from build123d import *

# Parameters (mm, degrees)
CUT_EXTRUDE_1_REACH = 10.022


with BuildPart() as part:
    # 草图1 → 旋转1 (revolve)
    with BuildSketch(Plane.XY, mode=Mode.PRIVATE) as revolve_1_sk:
        Polygon((1.5, -1.8), (1.5, -6.75), (1.25, -7), (0, -7), (0, -1.877350269), (1, -1.3), (1, 0), (2.77, 0), (2.77, -0.53), align=None)
    revolve(revolve_1_sk.sketch.rotate(Axis((0, 0, 0), (0, 1, 0)), 90), axis=Axis((0, 0, 0), (0, 1, 0)))

    # 切除-拉伸1: up to this cone (the profile starts inside it)
    cut_extrude_1_end = Plane(origin=(0, 0, 0), z_dir=(0, 1, 0)).offset(-1.877349269) * Cone(1.732e-06, 27.108355455, 15.651015319, align=(Align.CENTER, Align.CENTER, Align.MIN), mode=Mode.PRIVATE)
    # 草图2 → 切除-拉伸1 (cut, up to the surface)
    with BuildSketch(Plane(origin=(0, 0, 0), x_dir=(1, 0, 0), z_dir=(0, 1, 0)), mode=Mode.PRIVATE) as cut_extrude_1_sk1:
        Polygon((1.154700538, 0), (0.577350269, 1), (-0.577350269, 1), (-1.154700538, 0), (-0.577350269, -1), (0.577350269, -1), align=None)
    cut_extrude_1_tool1 = extrude(cut_extrude_1_sk1.sketch, amount=-CUT_EXTRUDE_1_REACH, mode=Mode.PRIVATE) & cut_extrude_1_end
    add(cut_extrude_1_tool1.solids().sort_by_distance((0, 0, 0))[0], mode=Mode.SUBTRACT)


solid = part.part
Source: CAD feature listing. Evaluate the final solid. Frame: model axes, mm. A direction names the side the tool comes from. Round coordinates to 2 decimals unless told otherwise and drop trailing zeros. Loops run counter-clockwise (first coordinate to the right, second up) from the corner with the lowest first, then second, coordinate; pieces in that order, holes last. Notation, with made-up numbers: (81, 47) -> (134, 47) arc R23 cw to (134, 57) -> close; hole circle Ø9 at (-23.5, 21.5). An arc over 180 degrees is marked (long way). Answer as a JSON object with one key per item and string values. Group by question number.
Q1. Contact query for flat-ended pins moving along their axis: P1, Ø3, axis at y = -6, z = 1, coming from the +X side; P2, Ø1, axis at x = 0, y = -3, coming from the +Z side; P3, Ø1.5, axis at y = -4, z = -1, coming from the -X side. Output: stop coordinate, or through.
Q2. Section query A-A (y = -0.25). Output: boundary loops of the cut face in (x, z).
Q3. Section query B-B (y = -3.5). Output: boundary loops of the cut face in (x, z).
Q4. Ray query, line 1 (X direction, y = -1.5, z = -0.25); line 2 (Y direction, x = -1.4, z = 1.45); line 3 (Z direction, x = 0.3, y = -0.5). Return the intervals inside material, ascending. Write a range as from..to.
Q5. Access query for faces 1 (the cylindrical face through (1.686, -0.269, 2.198)), 2 (the flat face through (0, -1, -1)). Directions: +Z, -Z, +X, -X, +Y, -Y. A direction counts if a zero-diameter tool reaches every point of the face in a straight line with its end or side. Return the directions, or none.
Q6. Section query C-C (y = -1.5). Output: boundary loops of the cut face in (x, z), plus the area to 3 significant figures.
Q7. Mould query, pull axis Z, two halves, no side actions, for faces 3 (the cylindrical face through (-0.45, -4.31, -1.43)), 4 (the flat face through (0.87, -0.64, -0.49)), 5 (the flat face through (0, 0, 1.2)). Classes: pulls with the +Z half, pulls with the -Z half, needs draft (parallel to the pull), parting line crosses it, or undercut.
Completed:
{
 "1": {"P1": "x = 1.5", "P2": "z = 1.5", "P3": "x = -1.48"},
 "2": {"outline": "circle Ø5.54 at (0, 0); hole (-1.15, 0) -> (-0.58, -1) -> (0.58, -1) -> (1.15, 0) -> (0.58, 1) -> (-0.58, 1) -> close"},
 "3": {"outline": "circle Ø3 at (0, 0)"},
 "4": {"line 1": "-1.78..-0.6, 0.6..1.78", "line 2": "-1.28..0", "line 3": "-2.75..-1, 1..2.75"},
 "5": {"face 1": "+Y, -Y", "face 2": "+Y"},
 "6": {"outline": "circle Ø3.6 at (0, 0); hole circle Ø1.31 at (0, 0)", "area": "8.84 mm²"},
 "7": {"face 3": "parting line crosses it", "face 4": "undercut", "face 5": "needs draft"}
}
